Geometry: final body of the model. Coordinates: model frame, mm. A direction names the side the tool comes from. Give positions to 0.01 mm unless a question says otherwise; leave off trailing zeros. Loops run counter-clockwise (first coordinate to the right, second up) from the corner with the lowest first, then second, coordinate; pieces in that order, holes last. Notation, with made-up numbers: (16.25, 72) -> (61.25, 72) arc R23 ccw to (61.25, 103) -> close; hole circle Ø7 at (21, 55.5). An arc over 180 degrees is marked (long way). Answer in a Markdown table with one row per item. Add a question column.
1) Draft query along Z for faces 1 (the cylindrical face through (7.243, 41.965, -0.128)), 2 (the flat face through (0, 19, -9.95)), 3 (the flat face through (-1, 38.5, 0)), 4 (the cylindrical face through (25.615, 26.507, -5.625)). Return one class per face: +Z half, -Z half, draft (parallel to the pull), parting line (faces both ways), or undercut.
2) Access query for faces 5 (the flat face through (24, 25.29, 0)), 6 (the flat face through (18, 36, -8)), 7 (the flat face through (-24, 25.29, 0)). Directions: +Z, -Z, +X, -X, +Y, -Y. A direction counts if a zero-diameter tool reaches every point of the face in a straight line with its end or side. Return the directions, or none.
3) Section query B-B (z = 5.75). Return the cut outline in (x, y), plus the area to 3 significant figures.
4) Section query A-A (x = 23.55). Return the cut outline in (y, z), plus the area to 3 significant figures.
5) Section query D-D (y = 33.5). Return the cut outline in (x, z), plus the area to 3 significant figures.
6) Section query C-C (x = -2.5). Return the cut outline in (y, z).
7) Line query: line 1 (Z direction, x = 23.55, y = 26.2); line 2 (X direction, y = 28, z = -5); line 3 (Y direction, x = -8, z = 7). Output: solid intervals per line, ascending. Write a range as from..to.
8) First-contact query: P1, Ø7, axis at x = 23.55, z = 4.975, coming from the +Y side; P2, Ø5, axis at x = -23.55, z = 4.975, coming from the -Y side; P3, Ø2, axis at y = 12.5, z = 6, coming from the -X side. Flat tips, straight axial feed; report the tip coordinate or a pass-through.
```python
from build123d import *

# Parameters (mm, degrees)
CROQUIS1_W              = 40.2
CROQUIS1_H              = 19.9
SALIENTE_EXTRUIR1_DEPTH = 36
CROQUIS4_W              = 19.9
CROQUIS4_H              = 2.4
SALIENTE_EXTRUIR3_DEPTH = 27
CROQUIS5_R              = 2.165
CORTAR_EXTRUIR2_DEPTH   = 57.31
SALIENTE_EXTRUIR5_DEPTH = 2.5
SALIENTE_EXTRUIR6_DEPTH = 1
CROQUIS8_R              = 2.91
SALIENTE_EXTRUIR7_DEPTH = 5
REDONDEO1_R             = 1


with BuildPart() as part:
    # Croquis1 → Saliente-Extruir1 (new body)
    with BuildSketch(Plane(origin=(0, 0, 0), x_dir=(1, 0, 0), z_dir=(0, 1, 0))):
        Rectangle(CROQUIS1_W, CROQUIS1_H)
    extrude(amount=SALIENTE_EXTRUIR1_DEPTH)

    # Croquis4 → Saliente-Extruir3 (add, symmetric)
    with BuildSketch(Plane(origin=(0, 0, 0), x_dir=(0, 0, -1), z_dir=(1, 0, 0))):
        with Locations((0, 26.49)):
            Rectangle(CROQUIS4_W, CROQUIS4_H)
    extrude(amount=SALIENTE_EXTRUIR3_DEPTH, both=True)

    # Croquis5 → Cortar-Extruir2 (cut)
    with BuildSketch(Plane(origin=(0, 27.69, 0), x_dir=(1, 0, 0), z_dir=(0, 1, 0))):
        with Locations((-23.55, 4.975)):
            Circle(CROQUIS5_R)
        with Locations((-23.55, -4.975)):
            Circle(CROQUIS5_R)
        with Locations((23.55, 4.975)):
            Circle(CROQUIS5_R)
        with Locations((23.55, -4.975)):
            Circle(CROQUIS5_R)
    extrude(amount=-CORTAR_EXTRUIR2_DEPTH, mode=Mode.SUBTRACT)

    # Croquis6 → Saliente-Extruir5 (add)
    with BuildSketch(Plane(origin=(0, 36, 0), x_dir=(1, 0, 0), z_dir=(0, 1, 0))):
        with BuildLine():
            ThreePointArc((10.15, -9.95), (0.2, 0), (10.15, 9.95))
            Line((10.15, 9.95), (-14.73, 9.95))
            Line((-14.73, 9.95), (-14.73, -9.95))
            Line((-14.73, -9.95), (10.15, -9.95))
        make_face()
        with BuildLine():
            ThreePointArc((20.1, 0), (17.185712473, 7.035712473), (10.15, 9.95))
            Line((10.15, 9.95), (10.15, -9.95))
            ThreePointArc((10.15, -9.95), (17.185712473, -7.035712473), (20.1, 0))
        make_face()
        with BuildLine():
            Line((10.15, -9.95), (10.15, 9.95))
            ThreePointArc((10.15, 9.95), (0.2, 0), (10.15, -9.95))
        make_face()
    extrude(amount=SALIENTE_EXTRUIR5_DEPTH)

    # Croquis7 → Saliente-Extruir6 (add)
    with BuildSketch(Plane(origin=(0, 38.5, 0), x_dir=(1, 0, 0), z_dir=(0, 1, 0))):
        with BuildLine():
            ThreePointArc((10.15, 6.5), (3.65, 0), (10.15, -6.5))
            Line((10.15, -6.5), (10.15, 6.5))
        make_face()
        with BuildLine():
            Line((10.15, 6.5), (10.15, -6.5))
            ThreePointArc((10.15, -6.5), (14.746194078, -4.596194078), (16.65, 0))
            ThreePointArc((16.65, 0), (14.746194078, 4.596194078), (10.15, 6.5))
        make_face()
    extrude(amount=SALIENTE_EXTRUIR6_DEPTH)

    # Croquis8 → Saliente-Extruir7 (add)
    with BuildSketch(Plane(origin=(0, 39.5, 0), x_dir=(1, 0, 0), z_dir=(0, 1, 0))):
        with Locations((10.15, 0)):
            Circle(CROQUIS8_R)
    extrude(amount=SALIENTE_EXTRUIR7_DEPTH)

    # Redondeo1
    redondeo1_edges = [part.edges().sort_by_distance(p)[0] for p in [
        (-27, 26.49, -9.95),
        (-27, 26.49, 9.95),
        (27, 26.49, -9.95),
        (27, 26.49, 9.95),
    ]]
    fillet(redondeo1_edges, radius=REDONDEO1_R)


solid = part.part
```
Evaluation:
| question | item | result |
|---|---|---|
| 1 | face 1 | parting line |
| 1 | face 2 | -Z half |
| 1 | face 3 | draft |
| 1 | face 4 | undercut |
| 2 | face 5 | +Z, -Z, +X, -Y |
| 2 | face 6 | -Z, +X, +Y |
| 2 | face 7 | +Z, -Z, -X, -Y |
| 3 | outline | (-27, 25.29) -> (-25.57, 25.29) -> (-25.57, 27.69) -> (-27, 27.69) -> close; (-21.53, 25.29) -> (-20.1, 25.29) -> (-20.1, 0) -> (20.1, 0) -> (20.1, 25.29) -> (21.53, 25.29) -> (21.53, 27.69) -> (20.1, 27.69) -> (20.1, 36) -> (18.27, 36) -> (18.27, 38.5) -> (13.18, 38.5) -> (13.18, 39.5) -> (7.12, 39.5) -> (7.12, 38.5) -> (-14.73, 38.5) -> (-14.73, 36) -> (-20.1, 36) -> (-20.1, 27.69) -> (-21.53, 27.69) -> close; (25.57, 25.29) -> (27, 25.29) -> (27, 27.69) -> (25.57, 27.69) -> close |
| 3 | area | 1,550 mm² |
| 4 | outline | (25.29, -9.95) -> (27.69, -9.95) -> (27.69, -7.14) -> (25.29, -7.14) -> close; (25.29, -2.81) -> (27.69, -2.81) -> (27.69, 2.81) -> (25.29, 2.81) -> close; (25.29, 7.14) -> (27.69, 7.14) -> (27.69, 9.95) -> (25.29, 9.95) -> close |
| 4 | area | 27.0 mm² |
| 5 | outline | (-20.1, -9.95) -> (20.1, -9.95) -> (20.1, 9.95) -> (-20.1, 9.95) -> close |
| 5 | area | 800 mm² |
| 6 | outline | (0, -9.95) -> (38.5, -9.95) -> (38.5, 9.95) -> (0, 9.95) -> close |
| 7 | line 1 | -9.95..-7.14, -2.81..2.81, 7.14..9.95 |
| 7 | line 2 | -20.1..20.1 |
| 7 | line 3 | 0..38.5 |
| 8 | P1 | y = 36 |
| 8 | P2 | y = 25.29 |
| 8 | P3 | x = -20.1 |
